from build123d import *

# Parameters (mm, degrees)
SKETCH1_W           = 60
SKETCH1_H           = 60
BOSS_EXTRUDE1_DEPTH = 20
SKETCH2_R           = 5
BOSS_EXTRUDE2_DEPTH = 25
SKETCH2_3_R         = 2
CUT_EXTRUDE1_DEPTH  = 89.459030065


with BuildPart() as part:
    # Sketch1 → Boss-Extrude1 (new body)
    with BuildSketch(Plane.XY):
        with Locations((-30, -30)):
            Rectangle(SKETCH1_W, SKETCH1_H)
    extrude(amount=BOSS_EXTRUDE1_DEPTH)

    # Sketch2 → Boss-Extrude2 (add)
    with BuildSketch(Plane.XY.offset(20)):
        with Locations(Location((-30, -14.599362292, 0), (0, 0, 180))):
            Circle(SKETCH2_R)
    extrude(amount=BOSS_EXTRUDE2_DEPTH)

    # Sketch2_3 → Cut-Extrude1 (cut, through all)
    with BuildSketch(Plane.XY.offset(20)):
        with Locations((-4, -4)):
            Circle(SKETCH2_3_R)
        with Locations((-4, -56)):
            Circle(SKETCH2_3_R)
        with Locations((-56, -4)):
            Circle(SKETCH2_3_R)
        with Locations((-56, -56)):
            Circle(SKETCH2_3_R)
    extrude(amount=-CUT_EXTRUDE1_DEPTH, mode=Mode.SUBTRACT)


solid = part.part
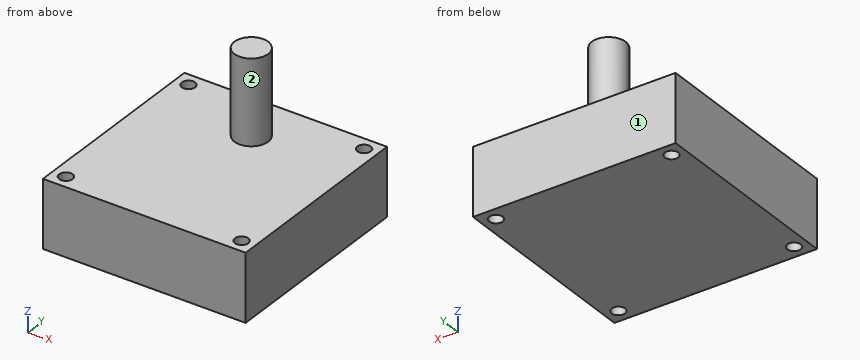
Design review of the part built by this model. Coordinates are the model's own, in mm. Face numbers are marked on the shaded views. A direction names the side the tool comes from. Coordinates: 2 decimals unless noted, no trailing zeros. Loops run counter-clockwise (first coordinate to the right, second up) from the corner with the lowest first, then second, coordinate; pieces in that order, holes last. Notation, with made-up numbers: (-4, -29.75) - (28, -29.75) arc R26 cw to (28, -15.75) - close; hole circle Ø9 at (26.25, 85). An arc over 180 degrees is marked (long way). Use CSV: the item, a comma, the result in double quotes. Start each with the question number.
1. For the marked faces 1 and 2, list the 3-axis set-ups (+Z, -Z, +X, -X, +Y, -Y) from which the entire face can be reached by the end or side of a thin tool; tool diameter is ignored.
2. Add section D-D on y = -17. Give the boundary of the cut face in (x, z), plus the area to 3 significant figures.
3. To check wall thickness, follow probe 1 along Y at (x, z) = (-56, 9.25); probe 2 along Z at (x, y) = (-12, -4.5); probe 3 along Y at (x, z) = (-26, 24.5). State the ranges of each line that lie inside material, in increasing order.
4. Add section A-A on y = -4. Give the boundary of the cut face in (x, z).
5. Clearance check with flat-ended pins moving along their axes: pin 1 (8 mm diameter, centred on x = -46.5, z = 27, fed in from -Y); pin 2 (3 mm diameter, centred on x = -17.5, y = -53, fed in from +Z); pin 3 (4 mm diameter, centred on x = -29, z = 8.5, fed in from +Y); pin 4 (6 mm diameter, centred on x = -26.5, z = 23.5, fed in from -Y). State where each tip first meets the part, or that it passes through.
6. Add section C-C on x = -30. Give the boundary of the cut face in (y, z).
Resolved:
1,face 1,"+Z, -Z, +X, -X, +Y"
1,face 2,"+Z"
2,outline,"(-60, 0) - (0, 0) - (0, 20) - (-25.61, 20) - (-25.61, 45) - (-34.39, 45) - (-34.39, 20) - (-60, 20) - close"
2,area,"1,420 mm2"
3,probe 1,"-60 to -58, -54 to -6, -2 to 0"
3,probe 2,"0 to 20"
3,probe 3,"-17.6 to -11.6"
4,outline,"(-60, 0) - (-58, 0) - (-58, 20) - (-60, 20) - close; (-54, 0) - (-6, 0) - (-6, 20) - (-54, 20) - close; (-2, 0) - (0, 0) - (0, 20) - (-2, 20) - close"
5,pin 1,"through"
5,pin 2,"z = 20"
5,pin 3,"y = 0"
5,pin 4,"y = -19.57"
6,outline,"(-60, 0) - (0, 0) - (0, 20) - (-9.6, 20) - (-9.6, 45) - (-19.6, 45) - (-19.6, 20) - (-60, 20) - close"
